Could you check a few things on this model? Use its own coordinates, in mm. A direction names the side the tool comes from. Give positions to 0.01 mm unless a question says otherwise; leave off trailing zeros. Order: outer loops, then holes, each group sorted by start corner. A loop starts at its lowest first (then second) coordinate and runs counter-clockwise, first axis right, second up.
(1) If I drill on probe 1 along Y at (x, z) = (-2, -5); probe 2 along Y at (x, z) = (-3.6, 0); probe 3 along Z at (x, y) = (-5.75, -1), over which ranges is the centre line in solid material (lowest first)?
(2) If we mould it in two halves opening along Y, with no side actions, what happens to faces 1 (the cylindrical face through (-9.46, -40.07, -86.16)), 2 (the cylindrical face through (-9.465, 54.544, 77.954)), 3 (the cylindrical face through (-4.228, -83.564, -18.556))? For each: released by +Y, released by -Y, zero draft, split by the parting line, or undercut.
(3) Imagine slicing it at A-A, the plane x = -4. Write out the boundary of the cut face in (y, z), then the cut area to 3 significant figures.
(4) On a 3-axis mill with a long thin cutter (end or side, diameter ignored), from which of +Z, -Z, +X, -X, +Y, -Y can I reach the whole of each face in a straight line? I mean faces 4 (the cylindrical face through (-9.465, 49.099, -89.464)), 5 (the cylindrical face through (-9.13, -15.62, -3.47)). Say none if no direction works.
(5) Imagine slicing it at B-B, the plane z = 0. State how many separate pieces and enclosed holes the cut face has, then the cut area to 3 significant figures.
(6) Will these pins go through, and if not, where does the flat tip stop? pin 1 (4 mm diameter, centred on x = -5.5, z = -69, fed in from -Y); pin 2 (4 mm diameter, centred on x = -4, y = -45.5, fed in from -Z); pin 3 (3.5 mm diameter, centred on y = -50, z = 86.6, fed in from -X) (3 decimals); pin 4 (5 mm diameter, centred on x = -9, z = -52.5, fed in from +Y).
from build123d import *

# Parameters (mm, degrees)
SKETCH2_R           = 92.875
SKETCH2_R_2         = 16
BOSS_EXTRUDE1_DEPTH = 5
SKETCH3_R           = 6
SKETCH3_R_2         = 3
BOSS_EXTRUDE2_DEPTH = 5
CIRPATTERN1_COUNT   = 6
BOSS_EXTRUDE3_START = -12
SKETCH4_R           = 16
SKETCH4_R_2         = 15
BOSS_EXTRUDE3_DEPTH = 1
FILLET1_R           = 0.2
CHAMFER1_SIZE       = 0.5
SKETCH5_R           = 88
SKETCH5_R_2         = 83
BOSS_EXTRUDE4_DEPTH = 5.8
CHAMFER2_SIZE       = 0.2
FILLET2_R           = 0.2
CUT_EXTRUDE1_START  = -0.8
SKETCH6_R           = 88
SKETCH6_R_2         = 85.6
CUT_EXTRUDE1_DEPTH  = 4


with BuildPart() as part:
    # Sketch2 → Boss-Extrude1 (new body)
    with BuildSketch(Plane.ZY.offset(7)):
        Circle(SKETCH2_R)
        Circle(SKETCH2_R_2, mode=Mode.SUBTRACT)
    extrude(amount=BOSS_EXTRUDE1_DEPTH)

    # Sketch3 → Boss-Extrude2 (add)
    with BuildSketch(Plane.ZY.offset(7)):
        with Locations((0, 100)):
            Circle(SKETCH3_R)
        with Locations((0, 100)):
            Circle(SKETCH3_R_2, mode=Mode.SUBTRACT)
        with BuildLine():
            ThreePointArc((-13.656930681, 91.865411714), (0, 92.875), (13.656930681, 91.865411714))
            ThreePointArc((13.656930681, 91.865411714), (8.317192306, 94.717589922), (5.992139168, 100.30703125))
            ThreePointArc((5.992139168, 100.30703125), (5.99803447, 100.153565931), (6, 100))
            ThreePointArc((6, 100), (-0.153565931, 94.00196553), (-5.992139168, 100.30703125))
            ThreePointArc((-5.992139168, 100.30703125), (-8.317192306, 94.717589922), (-13.656930681, 91.865411714))
        make_face()
    boss_extrude2 = extrude(amount=BOSS_EXTRUDE2_DEPTH)

    # CirPattern1: Boss-Extrude2 ×6 about axis
    cirpattern1_axis = Axis((0, 0, 0), (1, 0, 0))
    for i in range(1, CIRPATTERN1_COUNT):
        add(boss_extrude2.rotate(cirpattern1_axis, i * 360 / CIRPATTERN1_COUNT))

    # Sketch4 → Boss-Extrude3 (add)
    with BuildSketch(Plane(origin=(0, 0, 0), x_dir=(0, 0, -1), z_dir=(1, 0, 0)).offset(BOSS_EXTRUDE3_START)):
        Circle(SKETCH4_R)
        Circle(SKETCH4_R_2, mode=Mode.SUBTRACT)
    extrude(amount=BOSS_EXTRUDE3_DEPTH)

    # Fillet1
    fillet1_edges = [part.edges().sort_by_distance(p)[0] for p in [
        (-11, 0, -16),
    ]]
    fillet(fillet1_edges, radius=FILLET1_R)

    # Chamfer1
    chamfer1_edges = [part.edges().sort_by_distance(p)[0] for p in [
        (-7, 0, -16),
    ]]
    chamfer(chamfer1_edges, length=CHAMFER1_SIZE)

    # Sketch5 → Boss-Extrude4 (add)
    with BuildSketch(Plane.ZY.offset(7)):
        Circle(SKETCH5_R)
        Circle(SKETCH5_R_2, mode=Mode.SUBTRACT)
    extrude(amount=-BOSS_EXTRUDE4_DEPTH)

    # Chamfer2
    chamfer2_edges = [part.edges().sort_by_distance(p)[0] for p in [
        (-1.2, 0, -88),
        (-1.2, 0, -83),
    ]]
    chamfer(chamfer2_edges, length=CHAMFER2_SIZE)

    # Fillet2
    fillet2_edges = [part.edges().sort_by_distance(p)[0] for p in [
        (-7, 0, -83),
    ]]
    fillet(fillet2_edges, radius=FILLET2_R)

    # Sketch6 → Cut-Extrude1 (cut)
    with BuildSketch(Plane.ZY.offset(7).offset(CUT_EXTRUDE1_START)):
        Circle(SKETCH6_R)
        Circle(SKETCH6_R_2, mode=Mode.SUBTRACT)
    extrude(amount=-CUT_EXTRUDE1_DEPTH, mode=Mode.SUBTRACT)


solid = part.part
Answer block:
1. probe 1: y = -87.86 to -82.85, 82.85 to 87.86
1. probe 2: y = -85.6 to -83, 83 to 85.6
1. probe 3: z = -85.59 to -82.99, 82.99 to 85.59
2. face 1: undercut
2. face 2: released by +Y
2. face 3: split by the parting line
3. outline: circle Ø171.2 at (0, 0); hole circle Ø166 at (0, 0)
3. area: 1,380 mm2
4. face 4: +X, -X
4. face 5: +X
5. separate pieces: 4
5. enclosed holes: 0
5. area: 881 mm2
6. pin 1: stops at y = -63.6
6. pin 2: stops at z = -75.84
6. pin 3: passes through
6. pin 4: stops at y = 78.27
